Print and shaded views of the part. All mm, measured from the part's lowest x, y and z. A direction names the side the tool comes from. Give positions to 0.01 mm unless a question says otherwise; leave off trailing zeros. Loops run counter-clockwise (first coordinate to the right, second up) from the corner with the lowest first, then second, coordinate; pieces in that order, holes last. Notation, with made-up numbers: M 75.25,53 L 91.25,53 A36 cw 91.25,88 Z; hole C 10,-31 d4. An arc over 180 degrees is marked long. Answer in a Markdown table with one row per item.
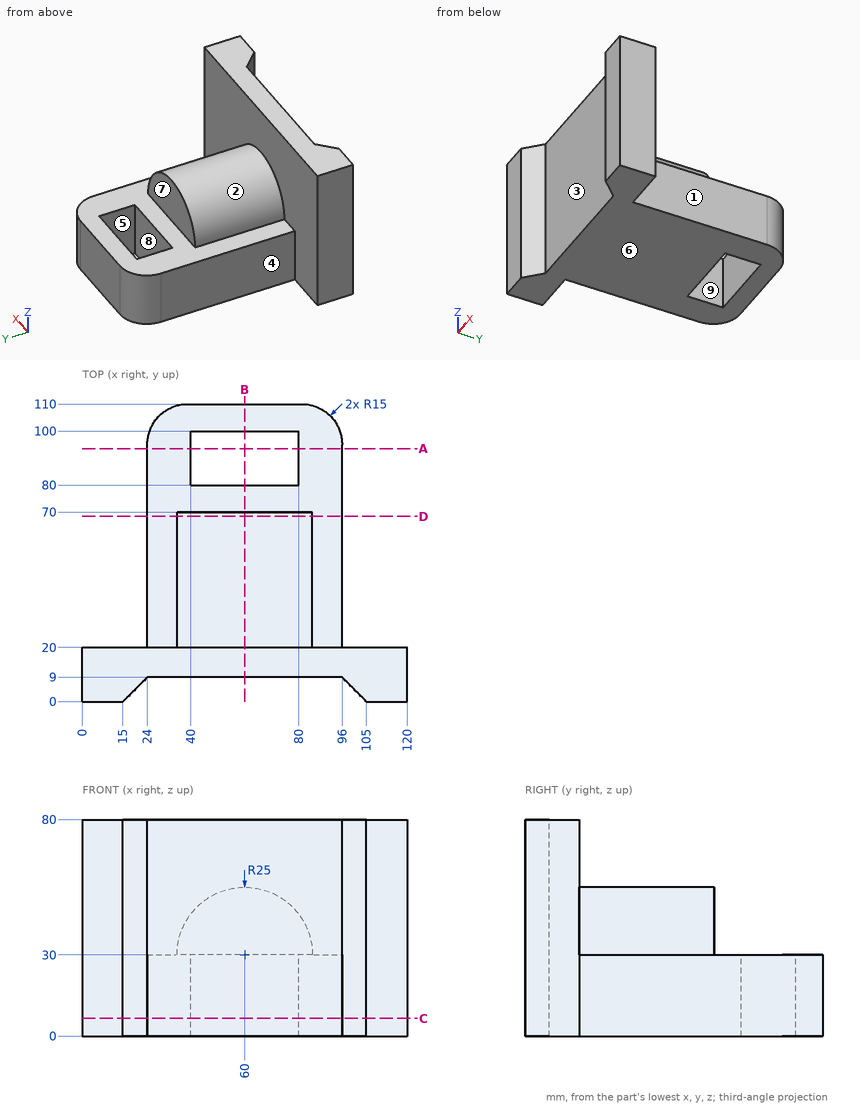
(1) Mould opens along Y. For the marked faces 6, 7, 8 and 9 say: pulls with the +Y half, pulls with the -Y half, needs draft (parallel to the pull), parting line crosses it, or undercut.
Established:
| item | result |
|---|---|
| face 6 | needs draft |
| face 7 | pulls with the +Y half |
| face 8 | undercut |
| face 9 | undercut |
(2) Saw through at B-B, the plane x = 60. Give the cut face in (y, z).
Established:
| item | result |
|---|---|
| outline | M 9,0 L 80,0 L 80,30 L 70,30 L 70,55 L 20,55 L 20,80 L 9,80 Z; M 100,0 L 110,0 L 110,30 L 100,30 Z |
(3) Which spindle directions (+Z, -Z, +X, -X, +Y, -Y) get a long thin tool onto all of the face, cutting with end or side? Do the marked faces 1, 2, 3, 4 and 5. Say none if no direction does.
Established:
| item | result |
|---|---|
| face 1 | +Z, -Z, +X, +Y |
| face 2 | +Z, +Y |
| face 3 | +Z, -Z, -Y |
| face 4 | +Z, -Z, -X, +Y |
| face 5 | +Z, -Z |
(4) Wall check: L1, parallel to Y at x = 56.5, z = 4; L2, parallel to Y at x = 50.5, z = 43; L3, parallel to X at y = 25.5, z = 13. Give the ranges that are in metal, low to high.
Established:
| item | result |
|---|---|
| L1 | y = 9 to 80, 100 to 110 |
| L2 | y = 9 to 70 |
| L3 | x = 24 to 96 |
(5) Saw through at D-D, the plane y = 68.5. Give the cut face in (x, z).
Established:
| item | result |
|---|---|
| outline | M 24,0 L 96,0 L 96,30 L 85,30 A25 ccw 35,30 L 24,30 Z |
(6) Saw through at C-C, the plane z = 6.5. Give the cut face in (x, y).
Established:
| item | result |
|---|---|
| outline | M 0,0 L 15,0 L 24,9 L 96,9 L 105,0 L 120,0 L 120,20 L 96,20 L 96,95 A15 ccw 81,110 L 39,110 A15 ccw 24,95 L 24,20 L 0,20 Z; hole M 40,80 L 80,80 L 80,100 L 40,100 Z |
(7) Flat gauge pins, fed straight in: P1, Ø20, axis at x = 54, z = 45.5, coming from the +Y side; P2, Ø10, axis at y = 89, z = 14.5, coming from the -X side; P3, Ø12, axis at y = 30, z = 35, coming from the +X side. Where does each tip first touch, or does it go through?
Established:
| item | result |
|---|---|
| P1 | stops at y = 70 |
| P2 | stops at x = 24 |
| P3 | stops at x = 96 |
(8) Saw through at A-A, the plane y = 93.5. Give the cut face in (x, z), and give its area (3 significant figures).
Established:
| item | result |
|---|---|
| outline | M 24,0 L 40,0 L 40,30 L 24,30 Z; M 80,0 L 96,0 L 96,30 L 80,30 Z |
| area | 960 mm2 |
